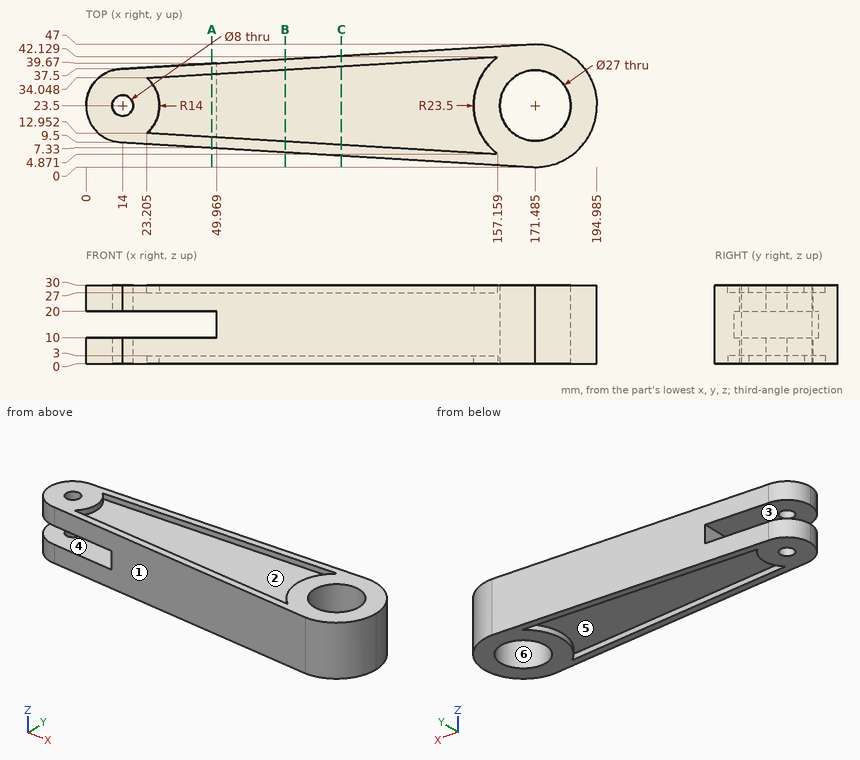
Study the drawing (mm; zero at the part's minimum x, y, z) and answer. A direction names the side the tool comes from. Give positions to 0.01 mm unless a question says otherwise; leave off trailing zeros. Write each loop counter-clockwise with the first axis right and the second up, starting at its lowest first coordinate (ties: lowest second). Pieces come first, ordered by that corner, then holes.
Item 1: Section C-C, the plane x = 97.5 is taken. Write down the section's boundary in (y, z), plus the area to 3 significant figures.
Item 2: Which of the six approach directions +Z, -Z, +X, -X, +Y, -Y give full straight-line access (tool end or side, diameter ignored) to the marked faces 4, 5 and 6?
Item 3: Determine the mould class of the marked faces 1, 2 and 3 for opening direction X: released by +X, released by -X, zero draft, split by the parting line, or undercut.
Item 4: Section A-A, the plane x = 48 is taken. Write down the section's boundary in (y, z).
Item 5: Find the intervals of material crossed by line 1 along Y through (x, z) = (14, 28); line 2 along X through (y, z) = (15, 2) (1 decimal); line 3 along X through (y, z) = (33, 27.5) (1 decimal), in increasing order.
Item 6: Section B-B, the plane x = 76 is taken. Write down the section's boundary in (y, z).
Item 7: Flat-ended cylindrical pins translate along their axes: P1, Ø1, axis at y = 16, z = 9, coming from the +X side; P2, Ø1, axis at y = 22, z = 20.5, coming from the -X side; P3, Ø8, axis at x = 169, y = 15, coming from the +Z side; P4, Ø4, axis at x = 52, y = 17, coming from the +Z side. Find the tip coordinate at first contact, or state that the pin passes through.
Completed:
1. outline: (4.46, 0) - (8.47, 0) - (8.47, 3) - (38.53, 3) - (38.53, 0) - (42.54, 0) - (42.54, 30) - (38.53, 30) - (38.53, 27) - (8.47, 27) - (8.47, 30) - (4.46, 30) - close
1. area: 962 mm2
2. face 4: -X, +Y, -Y
2. face 5: -Z
2. face 6: +Z, -Z
3. face 1: released by -X
3. face 2: undercut
3. face 3: zero draft
4. outline: (7.45, 0) - (11.46, 0) - (11.46, 3) - (35.54, 3) - (35.54, 0) - (39.55, 0) - (39.55, 10) - (7.45, 10) - close; (7.45, 20) - (39.55, 20) - (39.55, 30) - (35.54, 30) - (35.54, 27) - (11.46, 27) - (11.46, 30) - (7.45, 30) - close
5. line 1: y = 9.5 to 19.5, 27.5 to 37.5
5. line 2: x = 2.9 to 25.1, 149.6 to 161, 182 to 193.4
5. line 3: x = 3.7 to 24.3, 150 to 161.9, 181.1 to 193
6. outline: (5.76, 0) - (9.77, 0) - (9.77, 3) - (37.23, 3) - (37.23, 0) - (41.24, 0) - (41.24, 30) - (37.23, 30) - (37.23, 27) - (9.77, 27) - (9.77, 30) - (5.76, 30) - close
7. P1: stops at x = 193.92
7. P2: stops at x = 0.04
7. P3: passes through
7. P4: stops at z = 27
